Design review of the part built by this model. Coordinates are the model's own, in mm. A direction names the side the tool comes from. Coordinates: 2 decimals unless noted, no trailing zeros. Loops run counter-clockwise (first coordinate to the right, second up) from the corner with the lowest first, then second, coordinate; pieces in that order, holes last. Notation, with made-up numbers: (11, -35.5) - (32, -35.5) arc R25 cw to (32, -2.5) - close; hole circle Ø8 at (28.25, 37.5). An arc over 180 degrees is marked (long way). One line per question, with ' | ' between items.
from build123d import *

# Parameters (mm, degrees)
SKETCH1_W           = 140
SKETCH1_H           = 225
BOSS_EXTRUDE1_DEPTH = 10
CUT_EXTRUDE1_DEPTH  = 10
FILLET1_R           = 130
SKETCH3_W           = 10
SKETCH3_H           = 225
BOSS_EXTRUDE2_DEPTH = 15
SKETCH4_W           = 15
SKETCH4_H           = 31
CUT_EXTRUDE3_DEPTH  = 142.355049579


with BuildPart() as part:
    # Sketch1 → Boss-Extrude1 (new body)
    with BuildSketch(Plane.XY):
        Rectangle(SKETCH1_W, SKETCH1_H)
    extrude(amount=BOSS_EXTRUDE1_DEPTH)

    # Sketch2 → Cut-Extrude1 (cut)
    with BuildSketch(Plane.XY.offset(10)):
        with BuildLine():
            Line((70, 112.5), (-25, 112.5))
            add(Edge.make_bspline(
                [(-57, 12.829167661), (-57.230920503, 51.908636371), (-43.499555568, 87.434937954), (-25, 112.5)],
                knots=[0, 0, 0, 0, 1, 1, 1, 1], degree=3))
            Line((-57, 12.829167661), (70, -112.5))
            Line((70, -112.5), (70, 112.5))
        make_face()
        with BuildLine():
            Line((-57, 12.829167661), (70, -112.5))
            ThreePointArc((70, -112.5), (-15.444512377, -72.072482958), (-57, 12.829167661))
        make_face()
    extrude(amount=-CUT_EXTRUDE1_DEPTH, mode=Mode.SUBTRACT)

    # Fillet1
    fillet1_edges = [part.edges().sort_by_distance(p)[0] for p in [
        (-57, 12.829167661, 5),
    ]]
    fillet(fillet1_edges, radius=FILLET1_R)

    # Sketch3 → Boss-Extrude2 (add)
    with BuildSketch(Plane.ZY.offset(70)):
        with Locations((5, 0)):
            Rectangle(SKETCH3_W, SKETCH3_H)
    extrude(amount=BOSS_EXTRUDE2_DEPTH)

    # Sketch4 → Cut-Extrude3 (cut, through all)
    with BuildSketch(Plane(origin=(0, 0, 0), x_dir=(-1, 0, 0), z_dir=(0, 0, -1))):
        with Locations((77.5, 82.5)):
            Rectangle(SKETCH4_W, SKETCH4_H)
        with Locations((77.5, -72)):
            Rectangle(SKETCH4_W, SKETCH4_H)
    extrude(amount=-CUT_EXTRUDE3_DEPTH, mode=Mode.SUBTRACT)


solid = part.part
Q1. Draft analysis for pull direction Y (two halves, no side actions). For faces 3 (the flat face through (-77, -87.5, 5)), 4 (the flat face through (-53, -17, 10)), 5 (the flat face through (-77, 67, 5)), 6 (the flat face through (-6, -112.5, 5)), state which applies: +Y half, -Y half, draft (parallel to the pull), parting line (faces both ways), or undercut.
Returned:
face 3: undercut | face 4: draft | face 5: undercut | face 6: -Y half
Q2. Tool access review of faces 1 (the flat face through (-53, -17, 0)), 2 (the flat face through (-70, -72, 5)): name each direction out of +Z, -Z, +X, -X, +Y, -Y from which nothing blocks a thin tool from reaching the whole face with its end or side.
Returned:
face 1: -Z, +X, -X, +Y, -Y | face 2: +Z, -Z, -X
Q3. To check wall thickness, follow line 1 along Y through (x, z) = (-75, 6); line 2 along Y through (x, z) = (-28.5, 4); line 3 along Y through (x, z) = (-40, 6). State the ranges of each line that lie inside material, in increasing order.
Returned:
line 1: y = -112.5 to -87.5, -56.5 to 67, 98 to 112.5 | line 2: y = -112.5 to -57.28, 107.55 to 112.5 | line 3: y = -112.5 to -39.68, 87.54 to 112.5
Q4. Take a section at B-B (x = -14.5). Give the boundary of the cut face in (y, z), plus the area to 3 significant figures.
Returned:
outline: (-112.5, 0) - (-73, 0) - (-73, 10) - (-112.5, 10) - close | area: 395 mm²
Q5. For pin 1 (1.5 mm diameter, centred on y = -28.5, z = 9, fed in from +X); pin 2 (1 mm diameter, centred on y = 4.5, z = 5, fed in from +X), all flat-tipped, find the tip position at first contact; note any pin that passes through.
Returned:
pin 1: stops at x = -45.11 | pin 2: stops at x = -54.57
